```python
from build123d import *

# Parameters (mm, degrees)
F0_W     = 3
F0_H     = 20
F1_DEPTH = 3


with BuildPart() as f1:
    # F0 (on Front) → F1 (new body)
    with BuildSketch(Plane.XZ):
        Polygon((40, -38), (72, -38), (72, -10), (69, -10), (69, 10), (72, 10), (72, 38), (40, 38), (40, 35), (20, 35), (20, 38), (-20, 38), (-20, 35), (-40, 35), (-40, 38), (-72, 38), (-72, 10), (-69, 10), (-69, -10), (-72, -10), (-72, -38), (-40, -38), (-40, -35), (-20, -35), (-20, -38), (20, -38), (20, -35), (40, -35), align=None)
        Rectangle(F0_W, F0_H, mode=Mode.SUBTRACT)
    extrude(amount=F1_DEPTH)


solid = f1.part
```
Check sheet for the modelled part. Datum: model origin and axes. Units: mm. A direction names the side the tool comes from. Round coordinates to 2 decimals unless told otherwise and drop trailing zeros. Write each loop counter-clockwise with the first axis right and the second up, starting at its lowest first coordinate (ties: lowest second). Pieces come first, ordered by that corner, then holes. Notation, with made-up numbers: (-23, 44.25) -> (31, 44.25) arc R31 ccw to (31, 73.25) -> close; hole circle Ø5 at (14.5, 80.5). An arc over 180 degrees is marked (long way). One line per question, with ' | ' between items. Start each with the question number.
1. Sectioned sample at C-C, the plane x = -26.5. Record the cut outline in (y, z), then the cut area to 3 significant figures.
2. Release check for a two-part mould opening along Z. For faces 4 (the face through (-20, -1, 37)), 5 (the face through (0, -1, -10)), 6 (the face through (-30, -1, -35)) record: +Z half, -Z half, draft (parallel to the pull), parting line (faces both ways), or undercut.
3. Set-up check for faces 1 (the face through (-40, -1, -37)), 2 (the face through (1.5, -1, 0)), 3 (the face through (-40, -1, 36)): record each of +Z, -Z, +X, -X, +Y, -Y from which the full face is reachable in a straight line by a thin tool's end or side.
4. Sectioned sample at A-A, the plane z = 7. Record the cut outline in (x, y).
5. Scan lines: line 1 along X through (y, z) = (-0.9, 3.5); line 2 along Z through (x, y) = (-38.5, -0.7). Record each from-to range of solid material in increasing order. Write a range as from..to.
6. Depth check by flat-ended pin: pin 1 (0.9 mm diameter, centred on y = -1.5, z = 4.5, fed in from +X); pin 2 (3 mm diameter, centred on x = -16.5, z = -24.5, fed in from +Y); pin 3 (0.9 mm diameter, centred on y = -1.5, z = -3, fed in from -X); pin 4 (0.9 mm diameter, centred on x = 26, y = -2, fed in from -Z). Enter the tip coordinate at first touch or a pass-through.
Taken from the geometry:
1) outline: (-3, -35) -> (0, -35) -> (0, 35) -> (-3, 35) -> close | area: 210 mm^2
2) face 4: draft | face 5: undercut | face 6: -Z half
3) face 1: -Z, +Y, -Y | face 2: +Y, -Y | face 3: +Z, +Y, -Y
4) outline: (-69, -3) -> (-1.5, -3) -> (-1.5, 0) -> (-69, 0) -> close; (1.5, -3) -> (69, -3) -> (69, 0) -> (1.5, 0) -> close
5) line 1: x = -69..-1.5, 1.5..69 | line 2: z = -35..35
6) pin 1: stops at x = 69 | pin 2: stops at y = 0 | pin 3: stops at x = -69 | pin 4: stops at z = -35
